Part model, mm, in its own coordinate system. Face numbers are marked on the shaded views. A direction names the side the tool comes from. Give positions to 0.01 mm unless a question says otherwise; leave off trailing zeros. Order: outer loops, then holes, each group sorted by start corner. A loop starts at its lowest first (then second) coordinate and runs counter-clockwise, first axis right, second up. Notation, with made-up numbers: M 52.25,-39.5 L 82.25,-39.5 A6 ccw 82.25,-32.5 Z; hole C -30.75,-11 d7. An arc over 180 degrees is marked long. Return JSON: item names as keys, results as strings.
from build123d import *

# Parameters (mm, degrees)
EXTRUDE_1_DEPTH = 40
EXTRUDE_2_DEPTH = 4


with BuildPart() as part:
    # Sketch 1 → Extrude 1 (new body)
    with BuildSketch(Plane(origin=(0, 0, 0), x_dir=(1, 0, 0), z_dir=(0, 1, 0))):
        with BuildLine():
            Line((0, 40), (0, 0))
            Line((0, 0), (20, 0))
            Line((20, 0), (20, 14))
            ThreePointArc((20, 14), (14, 20), (20, 26))
            Line((20, 26), (20, 40))
            Line((20, 40), (0, 40))
        make_face()
        with BuildLine():
            ThreePointArc((20, 26), (14, 20), (20, 14))
            Line((20, 14), (20, 17.65))
            ThreePointArc((20, 17.65), (17.65, 20), (20, 22.35))
            Line((20, 22.35), (20, 26))
        make_face()
        with BuildLine():
            Line((20, 17.65), (20, 14))
            ThreePointArc((20, 14), (24.242640687, 15.757359313), (26, 20))
            ThreePointArc((26, 20), (24.242640687, 24.242640687), (20, 26))
            Line((20, 26), (20, 22.35))
            ThreePointArc((20, 22.35), (21.661700936, 21.661700936), (22.35, 20))
            ThreePointArc((22.35, 20), (21.661700936, 18.338299064), (20, 17.65))
        make_face()
        with BuildLine():
            Line((20, 14), (20, 0))
            Line((20, 0), (40, 0))
            Line((40, 0), (40, 40))
            Line((40, 40), (20, 40))
            Line((20, 40), (20, 26))
            ThreePointArc((20, 26), (24.242640687, 24.242640687), (26, 20))
            ThreePointArc((26, 20), (24.242640687, 15.757359313), (20, 14))
        make_face()
        with BuildLine():
            ThreePointArc((20, 22.35), (17.65, 20), (20, 17.65))
            Line((20, 17.65), (20, 19.1))
            ThreePointArc((20, 19.1), (19.1, 20), (20, 20.9))
            Line((20, 20.9), (20, 22.35))
        make_face()
        with BuildLine():
            Line((20, 19.1), (20, 17.65))
            ThreePointArc((20, 17.65), (21.661700936, 18.338299064), (22.35, 20))
            ThreePointArc((22.35, 20), (21.661700936, 21.661700936), (20, 22.35))
            Line((20, 22.35), (20, 20.9))
            ThreePointArc((20, 20.9), (20.636396103, 20.636396103), (20.9, 20))
            ThreePointArc((20.9, 20), (20.636396103, 19.363603897), (20, 19.1))
        make_face()
        with BuildLine():
            ThreePointArc((20, 20.9), (19.1, 20), (20, 19.1))
            Line((20, 19.1), (20, 20.9))
        make_face()
        with BuildLine():
            Line((20, 20.9), (20, 19.1))
            ThreePointArc((20, 19.1), (20.636396103, 19.363603897), (20.9, 20))
            ThreePointArc((20.9, 20), (20.636396103, 20.636396103), (20, 20.9))
        make_face()
    extrude(amount=-EXTRUDE_1_DEPTH)

    # Sketch 1_3 → Extrude 2 (add)
    with BuildSketch(Plane(origin=(0, 0, 0), x_dir=(1, 0, 0), z_dir=(0, 1, 0))):
        with BuildLine():
            ThreePointArc((20, 20.9), (19.1, 20), (20, 19.1))
            Line((20, 19.1), (20, 20.9))
        make_face()
        with BuildLine():
            Line((20, 20.9), (20, 19.1))
            ThreePointArc((20, 19.1), (20.636396103, 19.363603897), (20.9, 20))
            ThreePointArc((20.9, 20), (20.636396103, 20.636396103), (20, 20.9))
        make_face()
        with BuildLine():
            ThreePointArc((20, 26), (14, 20), (20, 14))
            Line((20, 14), (20, 17.65))
            ThreePointArc((20, 17.65), (17.65, 20), (20, 22.35))
            Line((20, 22.35), (20, 26))
        make_face()
        with BuildLine():
            Line((20, 17.65), (20, 14))
            ThreePointArc((20, 14), (24.242640687, 15.757359313), (26, 20))
            ThreePointArc((26, 20), (24.242640687, 24.242640687), (20, 26))
            Line((20, 26), (20, 22.35))
            ThreePointArc((20, 22.35), (21.661700936, 21.661700936), (22.35, 20))
            ThreePointArc((22.35, 20), (21.661700936, 18.338299064), (20, 17.65))
        make_face()
    extrude(amount=EXTRUDE_2_DEPTH)


solid = part.part
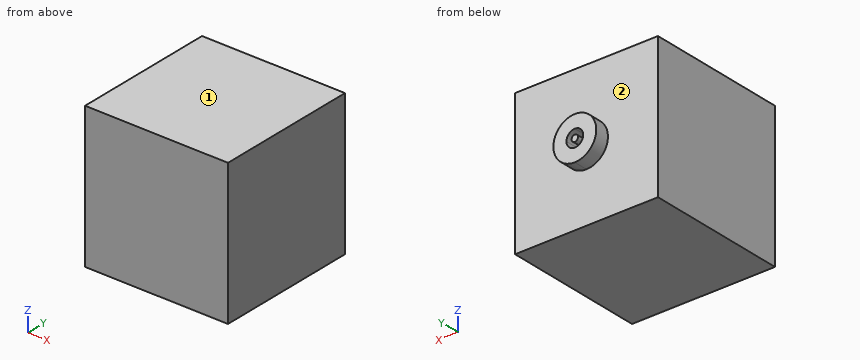
Q1. Band-saw the part on A-A (z = -5). Give the cut face in (x, y).
Established:
{"outline": "M 0,-40 L 40,-40 L 40,0 L 0,0 Z"}
Q2. Pin check, flat tip, straight feed: pin 1 (4 mm diameter, centred on x = 30, z = -25.5, fed in from +Y). Stop position of the tip, or through.
Established:
{"pin 1": "stops at y = 0"}
Q3. 3-axis set-ups, long thin cutter, end or side, ignore diameter. For the marked faces 1 and 2: which of +Z, -Z, +X, -X, +Y, -Y reach the whole face in a straight line?
Established:
{"face 1": "+Z, +X, -X, +Y, -Y", "face 2": "+Y"}
Q4. Probe line 1 along Y through (x, z) = (30, -5). List the from-to ranges inside material, lowest first.
Established:
{"line 1": "y = -40 to 0"}
Q5. Band-saw the part on B-B (x = 24). Give the cut face in (y, z), then the cut area to 3 significant figures.
Established:
{"outline": "M -40,-40 L 0,-40 L 0,-24.47 L 4,-24.47 L 4,-15.53 L 0,-15.53 L 0,0 L -40,0 Z", "area": "1,640 mm²"}
Q6. Band-saw the part on C-C (x = 29.5). Give the cut face in (y, z).
Established:
{"outline": "M -40,-40 L 0,-40 L 0,0 L -40,0 Z"}
